Geometry check sheet. Reference: the model listing, model coordinates, mm. A direction names the side the tool comes from. Coordinates: 2 decimals unless noted, no trailing zeros. Write each loop counter-clockwise with the first axis right and the second up, starting at its lowest first coordinate (ties: lowest second). Pieces come first, ordered by that corner, then holes. Notation, with made-up numbers: (62.25, -35.75) -> (98.25, -35.75) arc R20 cw to (98.25, -1.75) -> close; hole circle Ø2 at (-22, 53). An arc over 180 degrees is marked (long way). Use a Markdown table: item, result.
```python
from build123d import *

# Parameters (mm, degrees)
SKETCH1_W           = 30
SKETCH1_H           = 12
BOSS_EXTRUDE1_DEPTH = 3
SKETCH2_R           = 1.5
CUT_EXTRUDE1_DEPTH  = 4
CUT_EXTRUDE2_DEPTH  = 4
BOSS_EXTRUDE2_DEPTH = 3


with BuildPart() as part:
    # Sketch1 → Boss-Extrude1 (new body)
    with BuildSketch(Plane(origin=(0, 0, 0), x_dir=(1, 0, 0), z_dir=(0, 1, 0))):
        Rectangle(SKETCH1_W, SKETCH1_H)
    extrude(amount=BOSS_EXTRUDE1_DEPTH)

    # Sketch2 → Cut-Extrude1 (cut, through all)
    with BuildSketch(Plane(origin=(0, 3, 0), x_dir=(1, 0, 0), z_dir=(0, 1, 0))):
        with Locations((-9, 0)):
            Circle(SKETCH2_R)
        with Locations((9, 0)):
            Circle(SKETCH2_R)
    extrude(amount=-CUT_EXTRUDE1_DEPTH, mode=Mode.SUBTRACT)

    # Sketch3 → Cut-Extrude2 (cut, through all)
    with BuildSketch(Plane(origin=(0, 3, 0), x_dir=(1, 0, 0), z_dir=(0, 1, 0))):
        with BuildLine():
            Line((-6.5, 0), (-6.5, -6))
            ThreePointArc((-6.5, -6), (-9, -8.5), (-11.5, -6))
            Line((-11.5, -6), (-11.5, 0))
            ThreePointArc((-11.5, 0), (-9, 2.5), (-6.5, 0))
        make_face()
        with BuildLine():
            Line((11.5, 0), (11.5, -6))
            ThreePointArc((11.5, -6), (9, -8.5), (6.5, -6))
            Line((6.5, -6), (6.5, 0))
            ThreePointArc((6.5, 0), (9, 2.5), (11.5, 0))
        make_face()
    extrude(amount=-CUT_EXTRUDE2_DEPTH, mode=Mode.SUBTRACT)

    # Sketch4 → Boss-Extrude2 (add)
    with BuildSketch(Plane.XZ):
        with BuildLine():
            Line((-6, -6), (-6, 0))
            ThreePointArc((-6, 0), (0, 6), (6, 0))
            Line((6, 0), (6, -6))
            ThreePointArc((6, -6), (0, -12), (-6, -6))
        make_face()
    extrude(amount=-BOSS_EXTRUDE2_DEPTH)


solid = part.part
```
Item 1: Section check A-A on z = 1. Record the boundary of the cut face in (x, y), then the cut area to 3 significant figures.
Answer block:
| item | result |
|---|---|
| outline | (-15, 0) -> (-11.5, 0) -> (-11.5, 3) -> (-15, 3) -> close; (-6.5, 0) -> (6.5, 0) -> (6.5, 3) -> (-6.5, 3) -> close; (11.5, 0) -> (15, 0) -> (15, 3) -> (11.5, 3) -> close |
| area | 60.0 mm^2 |
Item 2: Section check B-B on y = 0.8. Record the boundary of the cut face in (x, z), then the cut area to 3 significant figures.
Answer block:
| item | result |
|---|---|
| outline | (-15, -6) -> (-6, -6) arc R6 ccw to (6, -6) -> (15, -6) -> (15, 6) -> (11.5, 6) -> (11.5, 0) arc R2.5 cw to (6.5, 0) -> (6.5, 6) -> (-6.5, 6) -> (-6.5, 0) arc R2.5 cw to (-11.5, 0) -> (-11.5, 6) -> (-15, 6) -> close |
| area | 337 mm^2 |
Item 3: Section check C-C on x = 9. Record the boundary of the cut face in (y, z), then the cut area to 3 significant figures.
Answer block:
| item | result |
|---|---|
| outline | (0, -6) -> (3, -6) -> (3, -2.5) -> (0, -2.5) -> close |
| area | 10.5 mm^2 |
Item 4: Section check D-D on z = -9.5. Record the boundary of the cut face in (x, y), then the cut area to 3 significant figures.
Answer block:
| item | result |
|---|---|
| outline | (-4.87, 0) -> (4.87, 0) -> (4.87, 3) -> (-4.87, 3) -> close |
| area | 29.2 mm^2 |
Item 5: Mould release check, pull along X, two halves, no side actions. Record for faces 4 (the flat face through (11.5, 2, 3)), 5 (the flat face through (-13, 1, 6)), 6 (the flat face through (15, 1, 0)): +X half, -X half, draft (parallel to the pull), parting line (faces both ways), or undercut.
Answer block:
| item | result |
|---|---|
| face 4 | undercut |
| face 5 | draft |
| face 6 | +X half |
Item 6: Tool access check on faces 1 (the flat face through (-11, 1, -6)), 2 (the flat face through (10, 1, -6)), 3 (the flat face through (-6.5, 2, 3)). Record the directions out of +Z, -Z, +X, -X, +Y, -Y that give a thin tool (end or side, any length) a straight path to the whole face; none if there is none.
Answer block:
| item | result |
|---|---|
| face 1 | -Z, -X, +Y, -Y |
| face 2 | -Z, +X, +Y, -Y |
| face 3 | +Z, +Y, -Y |
Item 7: Thickness scan on L1, parallel to X at y = 2.15, z = 1.25; L2, parallel to X at y = 2.75, z = -0.75; L3, parallel to Z at x = -11.75, y = 1.6. Record the ranges inside material, lowest first. Write a range as [from, to].
Answer block:
| item | result |
|---|---|
| L1 | x = [-15, -11.5], [-6.5, 6.5], [11.5, 15] |
| L2 | x = [-15, -11.38], [-6.62, 6.62], [11.38, 15] |
| L3 | z = [-6, 6] |
Item 8: Depth check by flat-ended pin: P1, Ø4, axis at x = 1, z = -8.5, coming from the -Y side. Enter the tip coordinate at first touch or a pass-through.
Answer block:
| item | result |
|---|---|
| P1 | stops at y = 0 |
